Input: dimensioned drawing with shaded views. Units: mm. Origin: part minimum x, y, z. Round coordinates to 2 decimals unless told otherwise and drop trailing zeros. Loops run counter-clockwise (first coordinate to the right, second up) from the corner with the lowest first, then second, coordinate; pieces in that order, holes last. Notation, with made-up numbers: (56, -34) - (115, -34) arc R14 cw to (115, -16) - close; hole circle Ø6 at (34, 12). An arc over 180 degrees is marked (long way). Answer as CSV lines item,"result".
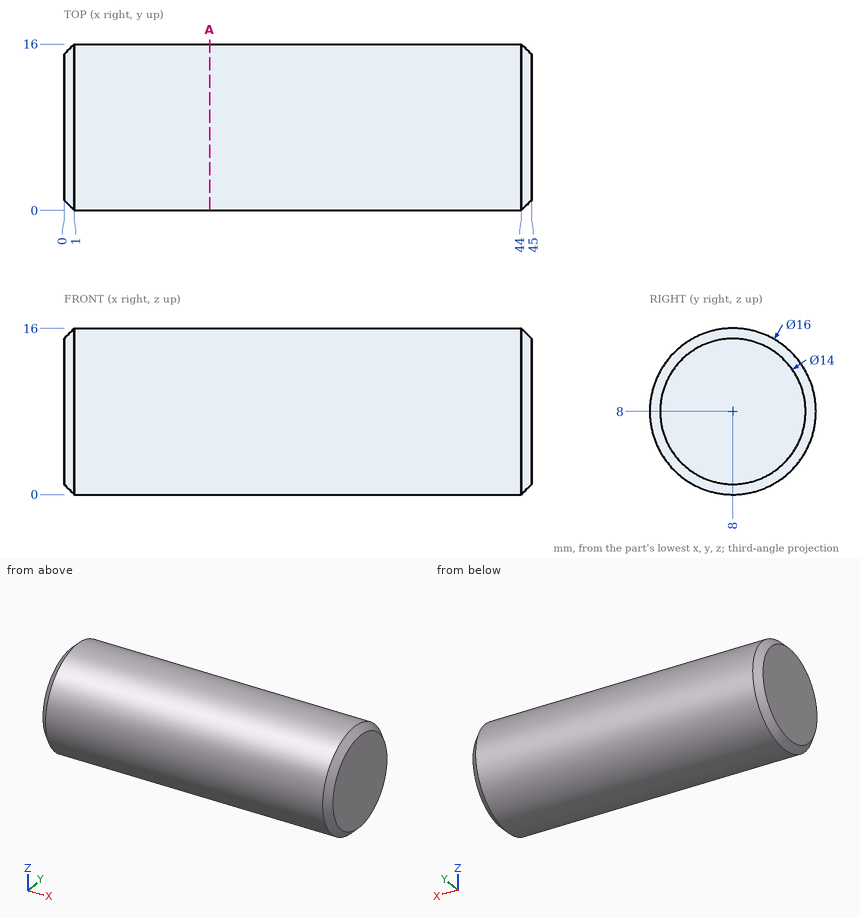
(1) Section A-A (x = 14). Output: boundary loops of the cut face in (y, z), and give its area (3 significant figures).
Findings below:
outline,"circle Ø16 at (8, 8)"
area,"201 mm2"
(2) Pin query (flat end, axial travel): P1, Ø3, axis at x = 39, z = 12, coming from the +Y side; P2, Ø1, axis at x = 20, z = 4, coming from the +Y side; P3, Ø1.5, axis at x = 31, z = 5, coming from the +Y side. Return the tip coordinate at first contact, or that it passes through.
Findings below:
P1,"y = 15.6"
P2,"y = 15.19"
P3,"y = 15.68"
(3) Material intervals for line 1 along Y through (x, z) = (32, 8.25); line 2 along Y through (x, z) = (31.5, 6); line 3 along Z through (x, y) = (19, 9.75), sorted ascending.
Findings below:
line 1,"0 to 16"
line 2,"0.25 to 15.75"
line 3,"0.19 to 15.81"
